```python
from build123d import *

# Parameters (mm, degrees)
F0_R     = 53.637742
F1_DEPTH = 92.44411
F3_ANGLE = 15
F4_ANGLE = 15


with BuildPart() as f1:
    # F0 (on Top) → F1 (new body)
    with BuildSketch(Plane.XY):
        Circle(F0_R)
    extrude(amount=F1_DEPTH)

    # F2 (on Front) → F3 (revolve)
    with BuildSketch(Plane.XZ):
        with BuildLine():
            Line((63.637742, 92.44411), (53.637742, 92.44411))
            Line((53.637742, 92.44411), (53.637742, 82.44411))
            ThreePointArc((53.637742, 82.44411), (56.566675, 89.515178), (63.637742, 92.44411))
        make_face()
    revolve(axis=Axis((0, 0, 0), (0, 0, -1)), revolution_arc=F3_ANGLE)

    # F2 (on Front) → F4 (revolve)
    with BuildSketch(Plane.XZ):
        Polygon((-63.637742, 82.44411), (-53.637742, 72.44411), (-53.637742, 92.44411), align=None)
    revolve(axis=Axis((0, 0, 0), (0, 0, -1)), revolution_arc=F4_ANGLE)


solid = f1.part
```
Input: part model. Units: mm. Frame: model coordinates. A direction names the side the tool comes from. Coordinates: 2 decimals unless noted, no trailing zeros. Loops run counter-clockwise (first coordinate to the right, second up) from the corner with the lowest first, then second, coordinate; pieces in that order, holes last. Notation, with made-up numbers: M 67,41.25 L 95,41.25 A29 cw 95,69.25 Z; hole C -7.5,62 d8. An arc over 180 degrees is marked long. Use a Markdown table: item, result. Add a question column.
1) Set-up query: faces 5 (the flat face through (56, 0, 90)), 6 (the flat face through (-1, 1, 0)), 7 (the flat face through (-58, 0, 83)). Return all of +Z, -Z, +X, -X, +Y, -Y with unobstructed straight access to the full face (end or side cutting, diameter ignored); none if empty.
2) Pin query (flat end, axial travel): P1, Ø4, axis at x = -42.5, z = 27.5, coming from the -Y side; P2, Ø3, axis at x = 36.5, z = 71, coming from the -Y side; P3, Ø1, axis at y = -9.5, z = 18, coming from the +X side. Return the tip coordinate at first contact, or that it passes through.
3) Section B-B, the plane x = 32.5. Return the cut outline in (y, z), plus the area to 3 significant figures.
4) Line query: L1, parallel to Y at x = -32, z = 89.5; L2, parallel to X at y = -37, z = 48; L3, parallel to Y at x = -42.5, z = 51. Output: solid intervals per line, ascending. Write a range as from..to.
5) Section C-C, the plane y = 42.5. Return the cut outline in (x, z), plus the area to 3 significant figures.
6) Draft query along X for faces 1 (the flat face through (53.755, -14.404, 90.06)), 2 (the conical face through (-58.219, 7.556, 87.374)), 3 (the flat face through (4, -1, 92.444)), 4 (the flat face through (-55.6, 14.9, 82.6)). Return one class per face: +X half, -X half, draft (parallel to the pull), parting line (faces both ways), or undercut.
7) Section D-D, the plane z = 12. Return the cut outline in (x, y).
8) Section A-A, the plane z = 85. Return the cut outline in (x, y), plus the area to 3 significant figures.
Answer below:
| question | item | result |
|---|---|---|
| 1 | face 5 | +Z, -Z, +X, +Y |
| 1 | face 6 | -Z, +X, -X, +Y, -Y |
| 1 | face 7 | +Z, -Z, -X, -Y |
| 2 | P1 | y = -35.17 |
| 2 | P2 | y = -40.64 |
| 2 | P3 | x = 52.88 |
| 3 | outline | M -42.67,0 L 42.67,0 L 42.67,92.44 L -42.67,92.44 Z |
| 3 | area | 7,890 mm2 |
| 4 | L1 | -43.05..43.05 |
| 4 | L2 | -38.83..38.83 |
| 4 | L3 | -32.72..32.72 |
| 5 | outline | M -32.72,0 L 32.72,0 L 32.72,92.44 L -32.72,92.44 Z |
| 5 | area | 6,050 mm2 |
| 6 | face 1 | undercut |
| 6 | face 2 | -X half |
| 6 | face 3 | draft |
| 6 | face 4 | undercut |
| 7 | outline | C 0,0 d107.28 |
| 8 | outline | M -61.08,0 L -53.64,0 A53.64 ccw 51.81,-13.88 L 52.13,-13.97 A53.97 ccw 53.97,0 L 53.64,0 A53.64 ccw -51.81,13.88 L -59,15.81 A61.08 ccw Z |
| 8 | area | 9,150 mm2 |
